The model under review builds one solid part; all positions refer to its coordinate system, in mm. A direction names the side the tool comes from. Give positions to 0.01 mm unless a question says otherwise; leave off trailing zeros. Loops run counter-clockwise (first coordinate to the right, second up) from the corner with the lowest first, then second, coordinate; pieces in that order, holes last. Notation, with made-up numbers: (0, -2) -> (38, -2) arc R18 cw to (38, 14) -> close; hole circle Ø8 at (11.5, -27). An arc over 180 degrees is marked (long way). Write each question's results on one line, items separated by ' | '. Start each with the question number.
Q1. We need section D-D (y = 0). Write out the cut boundary in (x, z), plus the area to 3 significant figures.
Q2. Mouldability with a two-part tool opening along X and no side actions: class faces 1 (the face through (63.899, -7, -6)), 2 (the face through (-70.431, 35, 13)), 3 (the face through (60.68, 1.24, -9.35)), 4 (the face through (-110.055, -7, -4)) as released by +X, released by -X, zero draft, split by the parting line, or undercut.
Q3. Machinability: for faces 5 (the face through (-70.431, -48, 13)), 6 (the face through (-30, 33, -58.13)), 7 (the face through (-24, -44.45, -24)), which of the approach directions +Z, -Z, +X, -X, +Y, -Y give a long, thin tool a straight path to every point of the face, cutting with its end or side? Answer none if there is none.
Q4. We need section B-B (x = -47). Write out the cut boundary in (y, z).
Q5. We need section C-C (z = 7). Write out the cut boundary in (x, y).
Q6. We need section A-A (y = 25.5). Write out the cut boundary in (x, z), plus the area to 3 significant figures.
Q7. Insertion check: pin 1 Ø3 at (x, y) = (-47, 34.5) entering from +Z. The pin has a flat end and moves straight along its axis. Give the tip position at first contact, or say it passes through.
Q8. Wall thickness on L1, parallel to Y at x = -50, z = -23; L2, parallel to X at y = -23, z = 8; L3, parallel to Z at x = 59, y = 0: over which ranges is each line inside the solid? List them lowest first. Write a range as [from, to].
from build123d import *

# Parameters (mm, degrees)
F1_DEPTH      = 50.8
F1_DEPTH_BACK = 38.1
F2_T          = -6.35
F4_D          = 19.05


with BuildPart() as f1:
    # F0 (on Front) → F1 (new body, two sides)
    with BuildSketch(Plane.XZ) as f1_sk:
        Polygon((-110.054575, 28.956002), (-110.054575, -58.129717), (63.899137, -58.129717), (63.899137, 28.956002), (20.138571, 28.956002), (20.138571, -3.265714), (-70.430569, -3.265714), (-70.430569, 28.956002), align=None)
    extrude(amount=F1_DEPTH)
    extrude(f1_sk.sketch, amount=-F1_DEPTH_BACK)

    # F2
    f2_openings = [f1.faces().sort_by_distance(p)[0] for p in [
        (-90.242572, -6.35, 28.956002),
        (-70.430569, -6.35, 12.845144),
        (20.138571, -6.35, 12.845144),
        (42.018854, -6.35, 28.956002),
        (-25.145999, -6.35, -3.265714),
        (-23.077719, -6.35, -58.129717),
    ]]
    offset(amount=F2_T, openings=f2_openings)

    # F4 (through all)
    with Locations(Plane.YZ.offset(63.899137)):
        with Locations((0, -18.793555)):
            Hole(F4_D / 2)


solid = f1.part
Output:
1) outline: (-110.05, -58.13) -> (-103.7, -58.13) -> (-103.7, -28.32) -> (-110.05, -28.32) -> close; (-110.05, -9.27) -> (-103.7, -9.27) -> (-103.7, 28.96) -> (-110.05, 28.96) -> close; (57.55, -58.13) -> (63.9, -58.13) -> (63.9, -28.32) -> (57.55, -28.32) -> close; (57.55, -9.27) -> (63.9, -9.27) -> (63.9, 28.96) -> (57.55, 28.96) -> close | area: 864 mm2
2) face 1: released by +X | face 2: undercut | face 3: zero draft | face 4: released by -X
3) face 5: +Z, +Y, -Y | face 6: -Z, +X, -X, +Y, -Y | face 7: +Z, -Z
4) outline: (-50.8, -58.13) -> (-44.45, -58.13) -> (-44.45, -3.27) -> (-50.8, -3.27) -> close; (31.75, -58.13) -> (38.1, -58.13) -> (38.1, -3.27) -> (31.75, -3.27) -> close
5) outline: (-110.05, -50.8) -> (-70.43, -50.8) -> (-70.43, -44.45) -> (-103.7, -44.45) -> (-103.7, 31.75) -> (-70.43, 31.75) -> (-70.43, 38.1) -> (-110.05, 38.1) -> close; (20.14, -50.8) -> (63.9, -50.8) -> (63.9, 38.1) -> (20.14, 38.1) -> (20.14, 31.75) -> (57.55, 31.75) -> (57.55, -44.45) -> (20.14, -44.45) -> close
6) outline: (-110.05, -58.13) -> (-103.7, -58.13) -> (-103.7, 28.96) -> (-110.05, 28.96) -> close; (57.55, -58.13) -> (63.9, -58.13) -> (63.9, 28.96) -> (57.55, 28.96) -> close | area: 1,110 mm2
7) pin 1: z = -3.27
8) L1: [-50.8, -44.45], [31.75, 38.1] | L2: [-110.05, -103.7], [57.55, 63.9] | L3: [-58.13, -28.32], [-9.27, 28.96]
